Source: CAD feature listing. Evaluate the final solid. Frame: model axes, mm. Coordinates: 2 decimals unless noted, no trailing zeros. Write each loop counter-clockwise with the first axis right and the second up, starting at its lowest first coordinate (ties: lowest second). Pieces come first, ordered by that corner, then holes. Notation, with made-up numbers: M 79,13 L 108,13 A28 cw 108,43 Z; hole C -35.75,-38.75 d10. An arc over 180 degrees is marked long. One line per item, written item: value. Start each with the question number.
Item 1: Pin query (flat end, axial travel): P1, Ø1, axis at x = -39, z = 43.5, coming from the -Y side; P2, Ø1, axis at x = -38, z = 33.5, coming from the +Y side; P3, Ø1, axis at x = -49, y = 19, coming from the -Z side. Return the tip coordinate at first contact, or that it passes through.
Item 2: Cut plane C-C, the plane x = -35. Output: boundary loops of the cut face in (y, z), then the cut area to 3 significant figures.
Item 3: Cut plane B-B, the plane x = -39.75. Output: boundary loops of the cut face in (y, z).
Item 4: Cut plane A-A, the plane y = 0. Output: boundary loops of the cut face in (x, z).
Item 5: Ray query, L1, parallel to Z at x = -38.5, y = 20.5; L2, parallel to Y at x = -35.5, z = -23.5; L3, parallel to Z at x = -39.5, y = 0. Return the intervals inside material, ascending. Write a range as from..to.
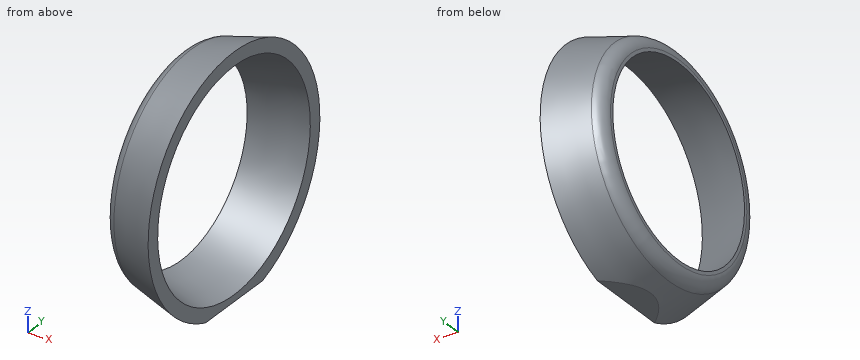
```python
from build123d import *

# Parameters (mm, degrees)
F2_W     = 50
F2_H     = 12.9609592259
F3_DEPTH = 35.1
F4_R     = 5


# Not quite as in the source:
# - a feature names something its author has since deleted; it is built from what else it names


with BuildPart() as f1:
    # F0 (on Front) → F1 (revolve)
    with BuildSketch(Plane.XZ):
        Polygon((-52.483901754, 46.9848437961), (-52.483901754, 41.9848437961), (-33.255017231, 47.4848437961), (-33.255017231, 52.4848437961), align=None)
    revolve(axis=Axis((-42.8694594925, 0, 7.4848437961), (1, 0, 0)))

    # F2 (on Front) → F3 (cut, symmetric)
    with BuildSketch(Plane.XZ):
        with Locations((-24.5732873678, -41.422042688)):
            Rectangle(F2_W, F2_H)
    extrude(amount=F3_DEPTH, both=True, mode=Mode.SUBTRACT)

    # F4
    f4_edges = [f1.edges().sort_by_distance(p)[0] for p in [
        (-52.483902, 0, -32.015156),
    ]]
    fillet(f4_edges, radius=F4_R)


solid = f1.part
```
From the geometry:
1. P1: stops at y = -24.91
1. P2: stops at y = 35.45
1. P3: stops at z = -28.59
2. outline: M -13.43,-34.94 L 13.43,-34.94 A44.5 ccw long Z; hole C 0,7.48 d79
2. area: 1,280 mm²
3. outline: M -7.83,-34.94 L 7.83,-34.94 A43.14 ccw long Z; hole C 0,7.48 d76.28
4. outline: M -52.48,-28.24 A5 ccw -48.86,-33.05 L -42.25,-34.94 L -33.26,-34.94 L -33.26,-32.52 L -52.48,-27.02 Z; M -52.48,41.98 L -33.26,47.48 L -33.26,52.48 L -48.86,48.02 A5 ccw -52.48,43.21 Z
5. L1: z = -30.88..-25.1, 40.07..45.85
5. L2: y = -31.74..-24.27, 24.27..31.74
5. L3: z = -34.94..-30.73, 45.7..50.7
